from build123d import *

# Parameters (mm, degrees)
F0_R     = 26.924
F1_DEPTH = 6.35
F2_R     = 31.75
F2_R_2   = 26.924
F3_DEPTH = 3.175
F4_R     = 4.762257
F5_DEPTH = 25.4
F6_R     = 1.27
F7_R     = 1.27
F8_R     = 0.254


with BuildPart() as f1:
    # F0 (on Top) → F1 (new body)
    with BuildSketch(Plane.XY):
        Circle(F0_R)
    extrude(amount=F1_DEPTH)

    # F2 (on face) → F3 (join)
    with BuildSketch(Plane.XY.offset(6.35)):
        Circle(F2_R)
        Circle(F2_R_2, mode=Mode.SUBTRACT)
        Circle(F2_R_2)
    extrude(amount=F3_DEPTH)

    # F4 (on face) → F5 (cut)
    with BuildSketch(Plane.XY.offset(9.525)):
        Circle(F4_R)
    extrude(amount=-F5_DEPTH, mode=Mode.SUBTRACT)

    # F6
    f6_edges = [f1.edges().sort_by_distance(p)[0] for p in [
        (-31.75, 0, 9.525),
    ]]
    fillet(f6_edges, radius=F6_R)

    # F7
    f7_edges = [f1.edges().sort_by_distance(p)[0] for p in [
        (-26.924, 0, 0),
    ]]
    fillet(f7_edges, radius=F7_R)

    # F8
    f8_edges = [f1.edges().sort_by_distance(p)[0] for p in [
        (-4.762257, 0, 9.525),
        (-25.654, 0, 0),
        (-4.762257, 0, 0),
    ]]
    fillet(f8_edges, radius=F8_R)


solid = f1.part
Here's how the part is built. I have some questions about the finished solid (model axes, mm). A direction names the side the tool comes from. Coordinates: 2 decimals unless noted, no trailing zeros. Order: outer loops, then holes, each group sorted by start corner. A loop starts at its lowest first (then second) coordinate and runs counter-clockwise, first axis right, second up.
Item 1: For faces 4 (the face through (-14.3, -23.4, 6.35)), 5 (the face through (-6.883, -30.995, 7.289)), which set-ups out of +Z, -Z, +X, -X, +Y, -Y let a thin tool reach every point of the face, with its end or its side?
Result sheet:
face 4: -Z
face 5: +Z, -Z
Item 2: I need wall thicknesses on line 1 (Y direction, x = 0, z = 5.25); line 2 (Y direction, x = 0, z = 7.25); line 3 (X direction, y = 4, z = 9.25). Which ranges of each line are inside material? Lowest first, please.
Result sheet:
line 1: y = -26.92 to -4.76, 4.76 to 26.92
line 2: y = -31.75 to -4.76, 4.76 to 31.75
line 3: x = -31.01 to -2.58, 2.58 to 31.01
Item 3: If we mould it in two halves opening along X, with no side actions, what happens to faces 1 (the face through (-21.37, -16.38, 3.77)), 2 (the face through (-0.62, 4.72, 4.83)), 3 (the face through (0, -6, 9.525))? For each: +X half, -X half, draft (parallel to the pull), parting line (faces both ways), or undercut.
Result sheet:
face 1: parting line
face 2: undercut
face 3: draft
Item 4: If we section it at C-C on z = 3: List the corners of the cut face in (x, y) for me.
Result sheet:
outline: circle Ø53.85 at (0, 0); hole circle Ø9.52 at (0, 0)
Item 5: For P1, Ø5, axis at y = -19, z = 6, coming from the -X side; P2, Ø5, axis at y = -2.5, z = 1.5, coming from the +X side; P3, Ø1, axis at x = -2.5, z = 1.5, coming from the -Y side; P4, Ø12, axis at x = 8, y = 24.5, coming from the -Z side, each with a flat end and sliding along its axis, tell me the tip position at first contact or that it passes through.
Result sheet:
P1: stops at x = -27.11
P2: stops at x = 26.92
P3: stops at y = -26.85
P4: stops at z = 0
Item 6: If we section it at A-A on x = 0: List the corners of the cut face in (y, z) for me (3 decimals).
Result sheet:
outline: (-31.75, 6.35) - (-26.924, 6.35) - (-26.924, 1.27) arc R1.27 ccw to (-25.654, 0) - (-5.016, 0) arc R0.254 ccw to (-4.762, 0.254) - (-4.762, 9.271) arc R0.254 ccw to (-5.016, 9.525) - (-30.48, 9.525) arc R1.27 ccw to (-31.75, 8.255) - close; (4.762, 0.254) arc R0.254 ccw to (5.016, 0) - (25.654, 0) arc R1.27 ccw to (26.924, 1.27) - (26.924, 6.35) - (31.75, 6.35) - (31.75, 8.255) arc R1.27 ccw to (30.48, 9.525) - (5.016, 9.525) arc R0.254 ccw to (4.762, 9.271) - close
